Work out the finished part from the listing and answer in its coordinate system (mm). Give positions to 0.01 mm unless a question says otherwise; leave off trailing zeros. Order: outer loops, then holes, each group sorted by start corner. A loop starts at its lowest first (then second) coordinate and runs counter-clockwise, first axis right, second up. Notation, with made-up numbers: (-34.5, 83) - (-3.5, 83) arc R20 cw to (-3.5, 99) - close; hole circle Ø10 at (-23.5, 88). An arc over 180 degrees is marked (long way). Put each result on its own line as item: value.
```python
from build123d import *

# Parameters (mm, degrees)
SKETCH_1_W         = 390
SKETCH_1_H         = 390
SKETCH_1_R         = 1.5
SKETCH_1_W_2       = 230
SKETCH_1_H_2       = 149
EXTRUDE_1081_DEPTH = 6


with BuildPart() as part:
    # 草图1 → Extrude 1081 (new body)
    with BuildSketch(Plane(origin=(0, 0, 0), x_dir=(1, 0, 0), z_dir=(0, 1, 0))):
        Rectangle(SKETCH_1_W, SKETCH_1_H)
        with Locations(Location((-110, 178.5, 0), (0, 0, 270))):
            Circle(SKETCH_1_R, mode=Mode.SUBTRACT)
        with Locations(Location((-110, 21.5, 0), (0, 0, 90))):
            Circle(SKETCH_1_R, mode=Mode.SUBTRACT)
        with Locations(Location((110, 21.5, 0), (0, 0, 270))):
            Circle(SKETCH_1_R, mode=Mode.SUBTRACT)
        with Locations(Location((110, 178.5, 0), (0, 0, 90))):
            Circle(SKETCH_1_R, mode=Mode.SUBTRACT)
        with Locations(Location((-185, 185, 0), (0, 0, 270))):
            Circle(SKETCH_1_R, mode=Mode.SUBTRACT)
        with Locations(Location((-185, -185, 0), (0, 0, 90))):
            Circle(SKETCH_1_R, mode=Mode.SUBTRACT)
        with Locations(Location((185, -185, 0), (0, 0, 270))):
            Circle(SKETCH_1_R, mode=Mode.SUBTRACT)
        with Locations(Location((185, 185, 0), (0, 0, 90))):
            Circle(SKETCH_1_R, mode=Mode.SUBTRACT)
        with Locations((0, 100)):
            Rectangle(SKETCH_1_W_2, SKETCH_1_H_2, mode=Mode.SUBTRACT)
        with BuildLine():
            Line((-50, -150), (50, -150))
            ThreePointArc((50, -150), (64.142135624, -144.142135624), (70, -130))
            Line((70, -130), (70, -50))
            Line((70, -50), (-70, -50))
            Line((-70, -50), (-70, -130))
            ThreePointArc((-70, -130), (-64.142135624, -144.142135624), (-50, -150))
        make_face(mode=Mode.SUBTRACT)
        Polygon((-165, -90), (-135, -30), (-105, -90), (-135, -70), align=None, mode=Mode.SUBTRACT)
        Polygon((105, -90), (135, -30), (165, -90), (135, -70), align=None, mode=Mode.SUBTRACT)
    extrude(amount=EXTRUDE_1081_DEPTH)


solid = part.part
```
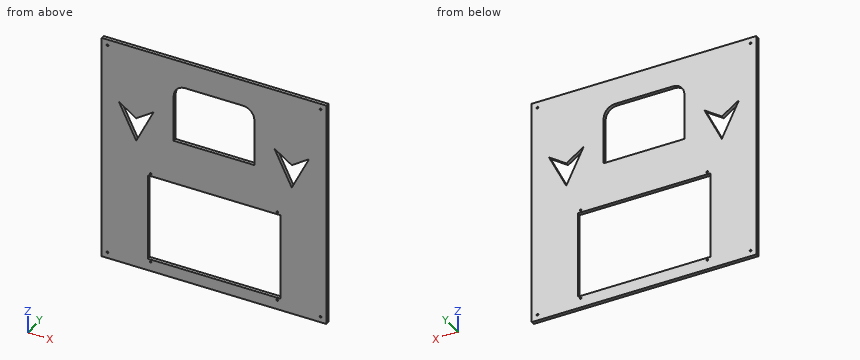
(1) Given pin 1 (1.8 mm diameter, centred on x = -185, z = -185, fed in from +Y); pin 2 (3.5 mm diameter, centred on x = 185, z = 185, fed in from -Y), each flat-ended and moving along its own axis, determine where each tip first touches the part or whether it passes through.
Geometry check:
pin 1: passes through
pin 2: stops at y = 0
(2) Section D-D, the plane x = 60 is taken. Write down the section's boundary in (y, z), then the cut area to 3 significant figures.
Geometry check:
outline: (0, -195) - (6, -195) - (6, -174.5) - (0, -174.5) - close; (0, -25.5) - (6, -25.5) - (6, 50) - (0, 50) - close; (0, 147.32) - (6, 147.32) - (6, 195) - (0, 195) - close
area: 862 mm²
(3) Straight lines are drawn through the part: line 1 (Z direction, x = -48, y = 2.8); line 2 (X direction, y = 1.8, z = -185); line 3 (Z direction, x = 98, y = 1.35). For each, find the intervals that lie inside material, in ascending order.
Geometry check:
line 1: z = -195 to -174.5, -25.5 to 50, 150 to 195
line 2: x = -195 to -186.5, -183.5 to 183.5, 186.5 to 195
line 3: z = -195 to -174.5, -25.5 to 195
(4) Section C-C, the plane y = 2 is taken. Count the separate pieces of the cut face and the enclosed holes in it, then the cut area to 3 significant figures.
Geometry check:
separate pieces: 1
enclosed holes: 12
area: 102,000 mm²
(5) Section B-B, the plane z = -157 is taken. Write down the section's boundary in (x, y).
Geometry check:
outline: (-195, 0) - (-115, 0) - (-115, 6) - (-195, 6) - close; (115, 0) - (195, 0) - (195, 6) - (115, 6) - close
(6) Section A-A, the plane x = -80.5 is taken. Write down the section's boundary in (y, z), then the cut area to 3 significant figures.
Geometry check:
outline: (0, -195) - (6, -195) - (6, -174.5) - (0, -174.5) - close; (0, -25.5) - (6, -25.5) - (6, 195) - (0, 195) - close
area: 1,450 mm²
